CAD build for the part. Positions are in the model's coordinates, mm. Face numbers are marked on the shaded views. Round coordinates to 2 decimals unless told otherwise and drop trailing zeros. Loops run counter-clockwise (first coordinate to the right, second up) from the corner with the lowest first, then second, coordinate; pieces in that order, holes last.
from build123d import *

# Parameters (mm, degrees)
SKETCH1_R           = 13
BOSS_EXTRUDE1_DEPTH = 44.45
CUT_EXTRUDE1_DEPTH  = 30.175
CHAMFER1_SIZE       = 1


with BuildPart() as part:
    # Sketch1 → Boss-Extrude1 (new body)
    with BuildSketch(Plane(origin=(0, 0, 0), x_dir=(1, 0, 0), z_dir=(0, 1, 0))):
        with BuildLine():
            Line((-14.5875, 0), (-14.5875, 19.7))
            Line((-14.5875, 19.7), (14.5875, 19.7))
            Line((14.5875, 19.7), (14.5875, 0))
            ThreePointArc((14.5875, 0), (0, -14.5875), (-14.5875, 0))
        make_face()
        Circle(SKETCH1_R, mode=Mode.SUBTRACT)
    extrude(amount=BOSS_EXTRUDE1_DEPTH)

    # Sketch3 → Cut-Extrude1 (cut, through all)
    with BuildSketch(Plane(origin=(14.5875, 0, 0), x_dir=(0, 0, -1), z_dir=(1, 0, 0))):
        Polygon((19.7, 30.1625), (18.1125, 30.1625), (18.1125, 31.75), (14.14375, 31.75), (14.14375, 18.25625), (18.1125, 18.25625), (18.1125, 19.84375), (19.7, 19.84375), align=None)
    extrude(amount=-CUT_EXTRUDE1_DEPTH, mode=Mode.SUBTRACT)

    # Chamfer1
    chamfer1_edges = [part.edges().sort_by_distance(p)[0] for p in [
        (0, 44.45, -19.7),
        (-14.5875, 44.45, -9.85),
        (-14.5875, 9.921875, -19.7),
        (14.5875, 9.921875, -19.7),
        (0, 44.45, 14.5875),
        (-14.5875, 0, -9.85),
        (0, 0, -19.7),
        (14.5875, 0, -9.85),
        (0, 0, 14.5875),
        (14.5875, 44.45, -9.85),
        (-14.5875, 37.30625, -19.7),
        (14.5875, 37.30625, -19.7),
    ]]
    chamfer(chamfer1_edges, length=CHAMFER1_SIZE)


solid = part.part
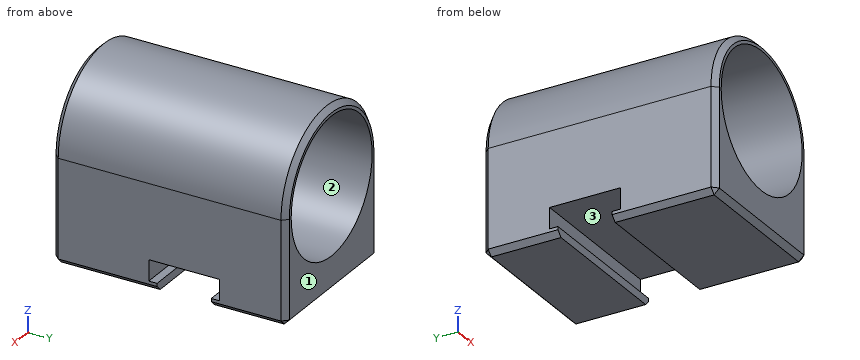
Item 1: Wall check: L1, parallel to Y at x = -1.75, z = -15.5; L2, parallel to Z at x = 0, y = 35; L3, parallel to Z at x = 0, y = 27. Give the ranges that are in metal, low to high.
Verdict:
L1: y = 0 to 18.26, 31.75 to 44.45
L2: z = -19.7 to -13, 13 to 14.59
L3: z = -14.14 to -13, 13 to 14.59
Item 2: Mould opens along Y. For the marked faces 1, 2 and 3 say: released by +Y, released by -Y, zero draft, split by the parting line, or undercut.
Verdict:
face 1: released by +Y
face 2: zero draft
face 3: undercut
Item 3: Cut at C-C (z = -3). List the corners of the cut face in (x, y).
Verdict:
outline: (-14.59, 1) - (-13.59, 0) - (-12.65, 0) - (-12.65, 44.45) - (-13.59, 44.45) - (-14.59, 43.45) - close; (12.65, 0) - (13.59, 0) - (14.59, 1) - (14.59, 43.45) - (13.59, 44.45) - (12.65, 44.45) - close
Item 4: Cut at A-A (x = 0). List the corners of the cut face in (y, z), plus the area to 3 significant figures.
Verdict:
outline: (0, -18.7) - (1, -19.7) - (19.84, -19.7) - (19.84, -18.11) - (18.26, -18.11) - (18.26, -14.14) - (31.75, -14.14) - (31.75, -18.11) - (30.16, -18.11) - (30.16, -19.7) - (43.45, -19.7) - (44.45, -18.7) - (44.45, -13) - (0, -13) - close; (0, 13) - (44.45, 13) - (44.45, 13.59) - (43.45, 14.59) - (1, 14.59) - (0, 13.59) - close
area: 296 mm2
Item 5: Flat gauge pins, fed straight in: P1, Ø1.5, axis at x = -3.5, y = 25, coming from the -Z side; P2, Ø1.7, axis at x = 2.5, y = 19, coming from the +Z side; P3, Ø1.3, axis at x = -5, y = 30.5, coming from the +Z side. Where does each tip first touch, or does it go through?
Verdict:
P1: stops at z = -14.14
P2: stops at z = 14.49
P3: stops at z = 13.92
Item 6: Cut at B-B (y = 4.5). List the corners of the cut face in (x, z) (1 decimal).
Verdict:
outline: (-14.6, -18.7) - (-13.6, -19.7) - (13.6, -19.7) - (14.6, -18.7) - (14.6, 0) arc R14.6 ccw to (-14.6, 0) - close; hole circle Ø26 at (0, 0)
